The model under review builds one solid part; all positions refer to its coordinate system, in mm. A direction names the side the tool comes from. Round coordinates to 2 decimals unless told otherwise and drop trailing zeros. Write each loop counter-clockwise with the first axis right and the second up, starting at its lowest first coordinate (ties: lowest second). Pieces come first, ordered by that corner, then holes.
Item 1: Add section B-B (y = 27). Give the boundary of the cut face in (x, z), plus the area to 3 significant figures.
Item 2: Add section D-D (y = -27). Give the boundary of the cut face in (x, z), plus the area to 3 significant figures.
Item 3: Add section A-A (x = 20.5). Give the boundary of the cut face in (y, z), plus the area to 3 significant figures.
Item 4: Add section C-C (z = 1.65). Give the boundary of the cut face in (x, y).
Item 5: To check wall thickness, follow L1, parallel to Y at x = 43, z = 2.75; L2, parallel to X at y = 41.5, z = 2.7; L3, parallel to Y at x = -75.5, z = 2.05. State the ranges of each line that lie inside material, in increasing order.
Item 6: Draft analysis for pull direction X (two halves, no side actions). For faces 4 (the face through (-85, -17, 1)), 5 (the face through (23, 24.5, 1)), 6 (the face through (-1, 1, 0)), state which applies: +X half, -X half, draft (parallel to the pull), parting line (faces both ways), or undercut.
Item 7: Clearance check with flat-ended pins moving along their axes: pin 1 Ø8 at (x, y) = (67, 19.5) entering from -Z; pin 2 Ø1.5 at (y, z) = (42.5, 2) entering from -X. State where each tip first meets the part, or that it passes through.
Item 8: Machinability: for faces 1 (the face through (85, -1, 1)), 2 (the face through (-80, 17, 1)), 3 (the face through (-31, -27, 1)), which of the approach directions +Z, -Z, +X, -X, +Y, -Y give a long, thin tool a straight path to every point of the face, cutting with its end or side? Answer none if there is none.
```python
from build123d import *

# Parameters (mm, degrees)
F1_DEPTH = 3


with BuildPart() as f1:
    # F0 (on Top) → F1 (new body)
    with BuildSketch(Plane.XY):
        Polygon((85, 52), (-75, 52), (-75, 17), (-85, 17), (-85, -52), (85, -52), align=None)
        with BuildLine():
            ThreePointArc((72.5, -24.5), (75, -27), (72.5, -29.5))
            Line((72.5, -29.5), (-28.5, -29.5))
            ThreePointArc((-28.5, -29.5), (-31, -27), (-28.5, -24.5))
            Line((-28.5, -24.5), (72.5, -24.5))
        make_face(mode=Mode.SUBTRACT)
        with BuildLine():
            Line((-28.5, 29.5), (72.5, 29.5))
            ThreePointArc((72.5, 29.5), (75, 27), (72.5, 24.5))
            Line((72.5, 24.5), (-28.5, 24.5))
            ThreePointArc((-28.5, 24.5), (-31, 27), (-28.5, 29.5))
        make_face(mode=Mode.SUBTRACT)
    extrude(amount=F1_DEPTH)


solid = f1.part
```
Numbers:
1. outline: (-75, 0) - (-31, 0) - (-31, 3) - (-75, 3) - close; (75, 0) - (85, 0) - (85, 3) - (75, 3) - close
1. area: 162 mm2
2. outline: (-85, 0) - (-31, 0) - (-31, 3) - (-85, 3) - close; (75, 0) - (85, 0) - (85, 3) - (75, 3) - close
2. area: 192 mm2
3. outline: (-52, 0) - (-29.5, 0) - (-29.5, 3) - (-52, 3) - close; (-24.5, 0) - (24.5, 0) - (24.5, 3) - (-24.5, 3) - close; (29.5, 0) - (52, 0) - (52, 3) - (29.5, 3) - close
3. area: 282 mm2
4. outline: (-85, -52) - (85, -52) - (85, 52) - (-75, 52) - (-75, 17) - (-85, 17) - close; hole (-28.5, -29.5) - (72.5, -29.5) arc R2.5 ccw to (72.5, -24.5) - (-28.5, -24.5) arc R2.5 ccw to start; hole (-28.5, 24.5) - (72.5, 24.5) arc R2.5 ccw to (72.5, 29.5) - (-28.5, 29.5) arc R2.5 ccw to start
5. L1: y = -52 to -29.5, -24.5 to 24.5, 29.5 to 52
5. L2: x = -75 to 85
5. L3: y = -52 to 17
6. face 4: -X half
6. face 5: undercut
6. face 6: draft
7. pin 1: stops at z = 0
7. pin 2: stops at x = -75
8. face 1: +Z, -Z, +X, +Y, -Y
8. face 2: +Z, -Z, -X, +Y
8. face 3: +Z, -Z
